Can you work these out from the model? Positions are in its coordinate system, mm. A direction names the side the tool comes from. Give positions to 0.01 mm unless a question says otherwise; leave off trailing zeros. Loops run counter-clockwise (first coordinate to the right, second up) from the corner with the lowest first, then second, coordinate; pieces in that order, holes last. Notation, with made-up numbers: (43, 28.25) - (95, 28.25) arc R11 ccw to (95, 42.25) - close; hole circle Ø1 at (22, 52). An arc over 180 degrees is marked (long way). Answer as a JSON object with one key per item and string values. Group by question number.
Item 1: Please list where these lines run through material, in increasing order: L1, parallel to X at y = 3, z = 0; L2, parallel to X at y = 7, z = 0; L3, parallel to X at y = 4, z = -43.5.
Item 2: Suppose I cut it at D-D on y = 34. Write out the boundary of the cut face in (x, z), and give its area (3 significant figures).
Item 3: Suppose I cut it at A-A on x = 30. Write out the boundary of the cut face in (y, z), and give its area (3 significant figures).
Item 4: Suppose I cut it at B-B on y = 17.5. Write out the boundary of the cut face in (x, z), and give its area (3 significant figures).
Item 5: Which directions (+Z, -Z, +X, -X, +Y, -Y) give clear straight access to the entire face, cutting with the end or side of a thin tool? Please do faces 4 (the cylindrical face through (13.124, 0.739, -3.86)), 5 (the flat face through (22, 6, -6.5)), 6 (the flat face through (-0.6, 8, 0)), 7 (the cylindrical face through (-1.98, 27.13, -41.75)).
Item 6: Suppose I cut it at C-C on y = -14.5. Write out the boundary of the cut face in (x, z).
Item 7: Will these pins go through, and if not, where does the flat tip stop? pin 1 (2.5 mm diameter, centred on y = 7, z = 0, fed in from -X); pin 2 (4 mm diameter, centred on y = 6.5, z = -28, fed in from +X); pin 3 (5 mm diameter, centred on x = 17, z = -9, fed in from -Y).
Item 8: Thinking about a two-plate mould opening in Y: for faces 1 (the flat face through (-21.998, 14, -42)), 2 (the flat face through (-16, -23.542, -42)), 3 (the cylindrical face through (-1.98, 30.78, -42.3)), which applies, pulls with the +Y half, pulls with the -Y half, needs draft (parallel to the pull), parting line crosses it, or undercut?
from build123d import *

# Parameters (mm, degrees)
BOSS_EXTRUDE1_DEPTH             = 5
SKETCH2_R                       = 1.75
SKETCH2_W                       = 10.8
SKETCH2_H                       = 10.8
CUT_EXTRUDE1_DEPTH              = 52.722948416
FILLET1_R                       = 5.4
FILLET2_R                       = 5.4
FILLET3_RADIUS                  = 10
FILLET3_LENGTH                  = 5
SKETCH3_W                       = 35
SKETCH3_H                       = 20
SKETCH3_W_2                     = 23
SKETCH3_H_2                     = 13
BOSS_EXTRUDE2_DEPTH             = 5.5
SKETCH4_W                       = 23
SKETCH4_H                       = 13
CUT_EXTRUDE2_DEPTH              = 3.5
CUT_EXTRUDE3_DEPTH              = 52.773674709
FILLET4_R                       = 4
SKETCH6_W                       = 8
SKETCH6_H                       = 28
BOSS_EXTRUDE3_DEPTH             = 32
FILLET5_R                       = 8
BOSS_EXTRUDE6_DEPTH             = 8
FILLET6_R                       = 4
SKETCH10_W                      = 5.3
SKETCH10_H                      = 13
SKETCH10_R                      = 1.4
BOSS_EXTRUDE7_DEPTH             = 9
BOSS_EXTRUDE8_START             = -10.5
BOSS_EXTRUDE8_DEPTH             = 10.5
SKETCH12_R                      = 1.35
CUT_EXTRUDE4_DEPTH              = 9
FILLET8_R                       = 5
SKETCH13_W                      = 4.9
SKETCH13_H                      = 13
CUT_EXTRUDE5_DEPTH              = 9
SKETCH14_R                      = 3
CUT_EXTRUDE6_DEPTH              = 71.938101594
FILLET10_R                      = 4
BOSS_EXTRUDE9_REACH             = 77.664
SKETCH15_R                      = 27
BOSS_EXTRUDE9_DIRECTION_2_DEPTH = 13
SKETCH17_R                      = 3
BOSS_EXTRUDE10_DEPTH            = 37.5
SKETCH18_R                      = 4
CUT_EXTRUDE7_DEPTH              = 2


# Some blends are built 0.0001 mm under size
with BuildPart() as part:
    # Sketch1 → Boss-Extrude1 (new body)
    with BuildSketch(Plane(origin=(0, 0, 0), x_dir=(1, 0, 0), z_dir=(0, 1, 0))):
        Polygon((45, -10), (45, 10), (21, 10), (11.001510114, 19.998489886), (-4.998489886, 19.998489886), (-14.999716743, 4.996611292), (-14.999716743, -10.003388708), (-4.998489886, -25.005267302), (11.001510114, -25.005267302), (20.99765203, -10), align=None)
    extrude(amount=BOSS_EXTRUDE1_DEPTH)

    # Sketch2 → Cut-Extrude1 (cut, through all)
    with BuildSketch(Plane(origin=(0, 5, 0), x_dir=(1, 0, 0), z_dir=(0, 1, 0))):
        with Locations(Location((-9.999716743, 0, 0), (0, 0, 270))):
            Circle(SKETCH2_R)
        with Locations(Location((-2.001032357, -20.005267302, 0), (0, 0, 270))):
            Circle(SKETCH2_R)
        with Locations(Location((7.998967643, -20.005267302, 0), (0, 0, 270))):
            Circle(SKETCH2_R)
        with Locations((16.9, 0)):
            Rectangle(SKETCH2_W, SKETCH2_H)
    extrude(amount=-CUT_EXTRUDE1_DEPTH, mode=Mode.SUBTRACT)

    # Fillet1
    fillet1_edges = [part.edges().sort_by_distance(p)[0] for p in [
        (11.5, 2.5, 5.4),
        (11.5, 2.5, -5.4),
    ]]
    fillet(fillet1_edges, radius=FILLET1_R - 0.0001)  # a hair under: the kernel refuses the full size

    # Fillet2
    # the kernel refuses this fillet: 5.4 mm, written as the material it adds along each edge
    with BuildSketch(Plane(origin=(22.3, 5, -5.4), x_dir=(0, 0, 1), z_dir=(0, -1, 0)), Plane(origin=(22.3, 5, 5.4), x_dir=(-1, 0, 0), z_dir=(0, -1, 0))) as fillet2_piece_1:
        with BuildLine():
            CenterArc((FILLET2_R, FILLET2_R), FILLET2_R, 180, 90)
            Line((0, FILLET2_R), (0, 0))
            Line((0, 0), (FILLET2_R, 0))
        make_face()
    extrude(amount=5)
    # the kernel refuses this fillet: 5.4 mm, written as the material it takes off along each edge

    # Fillet3: full round fillet: the end face becomes a half cylinder, R = half its width
    fillet3_face = Plane((45, 2.5, 0), x_dir=(0, 1, 0), z_dir=(1, 0, 0))  # on the end face: x along it, z out of the body
    fillet3_slab = fillet3_face.offset(-FILLET3_RADIUS / 2) * Box(FILLET3_LENGTH, 2 * FILLET3_RADIUS, FILLET3_RADIUS, mode=Mode.PRIVATE)  # the body's end, R deep
    fillet3_round = Plane((35, 2.5, 0), x_dir=(1, 0, 0), z_dir=(0, 1, 0)) * Cylinder(FILLET3_RADIUS, FILLET3_LENGTH, mode=Mode.PRIVATE)  # its axis R under the face
    add(fillet3_slab - fillet3_round, mode=Mode.SUBTRACT)

    # Sketch3 → Boss-Extrude2 (add)
    with BuildSketch(Plane(origin=(0, 5, 0), x_dir=(1, 0, 0), z_dir=(0, 1, 0))):
        with Locations((16.9, 0)):
            Rectangle(SKETCH3_W, SKETCH3_H)
        with Locations((16.9, 0)):
            Rectangle(SKETCH3_W_2, SKETCH3_H_2, mode=Mode.SUBTRACT)
    extrude(amount=BOSS_EXTRUDE2_DEPTH)

    # Sketch4 → Cut-Extrude2 (cut)
    with BuildSketch(Plane(origin=(0, 5, 0), x_dir=(1, 0, 0), z_dir=(0, 1, 0))):
        with Locations((16.9, 0)):
            Rectangle(SKETCH4_W, SKETCH4_H)
    extrude(amount=-CUT_EXTRUDE2_DEPTH, mode=Mode.SUBTRACT)

    # Sketch5 → Cut-Extrude3 (cut, through all)
    with BuildSketch(Plane(origin=(0, 5, 0), x_dir=(1, 0, 0), z_dir=(0, 1, 0))):
        with BuildLine():
            Line((34.4, 10), (34.4, -10))
            Line((34.4, -10), (35, -10))
            ThreePointArc((35, -10), (45, 0), (35, 10))
            Line((35, 10), (34.4, 10))
        make_face()
    extrude(amount=-CUT_EXTRUDE3_DEPTH, mode=Mode.SUBTRACT)

    # Fillet4
    fillet4_edges = [part.edges().sort_by_distance(p)[0] for p in [
        (34.4, 5.25, 10),
        (34.4, 5.25, -10),
    ]]
    fillet(fillet4_edges, radius=FILLET4_R)

    # Sketch6 → Boss-Extrude3 (add)
    with BuildSketch(Plane(origin=(0, 0, -19.998489886), x_dir=(-1, 0, 0), z_dir=(0, 0, -1))):
        with Locations((4.998489886, 14)):
            Rectangle(SKETCH6_W, SKETCH6_H)
    extrude(amount=BOSS_EXTRUDE3_DEPTH)

    # Fillet5
    fillet5_edges = [part.edges().sort_by_distance(p)[0] for p in [
        (-4.998489886, 0, -51.998489886),
        (-4.998489886, 28, -51.998489886),
    ]]
    fillet(fillet5_edges, radius=FILLET5_R)

    # Sketch9 → Boss-Extrude6 (add)
    with BuildSketch(Plane.ZY.offset(8.998489886)):
        Polygon((-10, 10.5), (-19.998489886, 28), (-19.998489886, 0), (-10, 0), align=None)
    extrude(amount=-BOSS_EXTRUDE6_DEPTH)

    # Fillet6
    fillet6_edges = [part.edges().sort_by_distance(p)[0] for p in [
        (-0.998489886, 2.5, -19.998489886),
        (20.99765203, 2.5, 10),
        (11.001510114, 2.5, 25.005267302),
        (-4.998489886, 2.5, 25.005267302),
        (-14.999716743, 2.5, 10.003388708),
        (-14.999716743, 2.5, -4.996611292),
        (11.001510114, 2.5, -19.998489886),
        (21, 2.5, -10),
        (-8.998489886, 2.5, -13.998474565),
    ]]
    fillet(fillet6_edges, radius=FILLET6_R)

    # Sketch10 → Boss-Extrude7 (add)
    with BuildSketch(Plane(origin=(0, 1.5, 0), x_dir=(1, 0, 0), z_dir=(0, 1, 0))):
        with Locations((8.05, 0)):
            Rectangle(SKETCH10_W, SKETCH10_H)
        with Locations(Location((8.05, 0, 0), (0, 0, 90))):
            Circle(SKETCH10_R, mode=Mode.SUBTRACT)
    extrude(amount=BOSS_EXTRUDE7_DEPTH)

    # Sketch11 → Boss-Extrude8 (add)
    with BuildSketch(Plane(origin=(0, 10.5, 0), x_dir=(1, 0, 0), z_dir=(0, 1, 0)).offset(BOSS_EXTRUDE8_START)):
        with BuildLine():
            Line((30.4, 10), (38.3, 10))
            Line((38.3, 10), (38.3, -10))
            Line((38.3, -10), (30.4, -10))
            ThreePointArc((30.4, -10), (33.228427125, -8.828427125), (34.4, -6))
            Line((34.4, -6), (34.4, 6))
            ThreePointArc((34.4, 6), (33.228427125, 8.828427125), (30.4, 10))
        make_face()
    extrude(amount=BOSS_EXTRUDE8_DEPTH)

    # Sketch12 → Cut-Extrude4 (cut)
    with BuildSketch(Plane(origin=(0, 10.5, 0), x_dir=(1, 0, 0), z_dir=(0, 1, 0))):
        with Locations(Location((35.65, 0, 0), (0, 0, 270))):
            Circle(SKETCH12_R)
    extrude(amount=-CUT_EXTRUDE4_DEPTH, mode=Mode.SUBTRACT)

    # Fillet8
    fillet8_edges = [part.edges().sort_by_distance(p)[0] for p in [
        (38.3, 5.25, -10),
        (38.3, 5.25, 10),
    ]]
    fillet(fillet8_edges, radius=FILLET8_R)

    # Sketch13 → Cut-Extrude5 (cut)
    with BuildSketch(Plane(origin=(0, 10.5, 0), x_dir=(1, 0, 0), z_dir=(0, 1, 0))):
        with Locations((30.85, 0)):
            Rectangle(SKETCH13_W, SKETCH13_H)
    extrude(amount=-CUT_EXTRUDE5_DEPTH, mode=Mode.SUBTRACT)

    # Sketch14 → Cut-Extrude6 (cut, through all)
    with BuildSketch(Plane(origin=(-0.998489886, 0, 0), x_dir=(0, 0, -1), z_dir=(1, 0, 0))):
        with Locations((41, 22)):
            Circle(SKETCH14_R)
        with Locations((41, 6)):
            Circle(SKETCH14_R)
    extrude(amount=-CUT_EXTRUDE6_DEPTH, mode=Mode.SUBTRACT)

    # Fillet10
    fillet10_edges = [part.edges().sort_by_distance(p)[0] for p in [
        (-4.998489886, 28, -19.998489886),
    ]]
    fillet(fillet10_edges, radius=FILLET10_R)

    # Boss-Extrude9: up to this face of the body (flat: up to its plane)
    boss_extrude9_end = Plane(part.part.faces().sort_by_distance((-0.998489886, 14.084187899, -32.543371898))[0])
    # Sketch15 → Boss-Extrude9 (add, up to the picked face)
    with BuildSketch(Plane.ZY.offset(8.998489886), mode=Mode.PRIVATE) as boss_extrude9_sk1:
        with Locations(Location((-41.998489886, 13.958456326, 0), (0, 0, 328.870116099))):
            Circle(SKETCH15_R)
    boss_extrude9_tool1 = split(extrude(boss_extrude9_sk1.sketch, amount=-BOSS_EXTRUDE9_REACH, mode=Mode.PRIVATE), bisect_by=boss_extrude9_end, keep=Keep.BOTH, mode=Mode.PRIVATE)
    add(boss_extrude9_tool1.solids().sort_by(Axis((-8.99849, 13.958456, -41.99849), (1, 0, 0)))[0])

    # Sketch15 → Boss-Extrude9 direction 2 (add)
    with BuildSketch(Plane.ZY.offset(8.998489886)):
        with Locations(Location((-41.998489886, 13.958456326, 0), (0, 0, 328.870116099))):
            Circle(SKETCH15_R)
    extrude(amount=BOSS_EXTRUDE9_DIRECTION_2_DEPTH)

    # Sketch17 → Boss-Extrude10 (add, symmetric)
    with BuildSketch(Plane(origin=(0, 13.958456326, 0), x_dir=(1, 0, 0), z_dir=(0, 1, 0))):
        with Locations(Location((-15.998489886, 41.998489886, 0), (0, 0, 90))):
            Circle(SKETCH17_R)
    extrude(amount=BOSS_EXTRUDE10_DEPTH, both=True)

    # Sketch18 → Cut-Extrude7 (cut)
    with BuildSketch(Plane(origin=(-0.998489886, 0, 0), x_dir=(0, 0, -1), z_dir=(1, 0, 0))):
        with Locations((53.998489886, 7.958456326)):
            Circle(SKETCH18_R)
        with Locations((29.998489886, 7.958456326)):
            Circle(SKETCH18_R)
        with BuildLine():
            ThreePointArc((55.430471337, 21.482233331), (42.06121766, 30.791596739), (28.086871666, 22.41789714))
            ThreePointArc((28.086871666, 22.41789714), (28.923742357, 19.962632481), (31.379007016, 20.799503173))
            ThreePointArc((31.379007016, 20.799503173), (41.935762112, 27.125315913), (52.035407344, 20.092666969))
            ThreePointArc((52.035407344, 20.092666969), (54.427722522, 19.089918153), (55.430471337, 21.482233331))
        make_face()
    extrude(amount=-CUT_EXTRUDE7_DEPTH, mode=Mode.SUBTRACT)


solid = part.part
Worked out:
{
 "1": {"L1": "x = -15 to -11.75, -8.25 to 6.65, 9.45 to 10.7, 33.3 to 34.3, 37 to 38.3", "L2": "x = -0.6 to 6.65, 9.45 to 10.7, 33.3 to 34.3, 37 to 38.3", "L3": "x = -22 to -1"},
 "2": {"outline": "(-22, -60.09) - (-1, -60.09) - (-1, -23.91) - (-22, -23.91) - close", "area": "760 mm2"},
 "3": {"outline": "(0, -10) - (10.5, -10) - (10.5, -6.5) - (1.5, -6.5) - (1.5, 6.5) - (10.5, 6.5) - (10.5, 10) - (0, 10) - close", "area": "93.0 mm2"},
 "4": {"outline": "(-22, -68.77) - (-1, -68.77) - (-1, -14) - (-9, -14) - (-9, -15.23) - (-22, -15.23) - close", "area": "1,130 mm2"},
 "5": {"face 4": "+Y, -Y", "face 5": "+Y", "face 6": "+Z, -Z, -X, +Y", "face 7": "+X"},
 "6": {"outline": "circle Ø6 at (-16, -42)"},
 "7": {"pin 1": "stops at x = -0.6", "pin 2": "stops at x = -1", "pin 3": "stops at y = 0"},
 "8": {"face 1": "needs draft", "face 2": "pulls with the -Y half", "face 3": "undercut"}
}
